For this review, take the finished solid that the model builds, in its own axes (mm). A direction names the side the tool comes from. Give positions to 0.01 mm unless a question says otherwise; leave off trailing zeros. Order: outer loops, then holes, each group sorted by start corner. A loop starts at its lowest first (then second) coordinate and runs counter-clockwise, first axis right, second up. Notation, with made-up numbers: (-6, 44) -> (12, 44) arc R16 ccw to (12, 65) -> close; hole circle Ø1 at (-18.75, 0.25). An arc over 180 degrees is marked (long way). Return JSON: item names as keys, results as strings. Group by question number.
1) Add section B-B (z = -94.5). Give the boundary of the cut face in (x, y), then the cut area to 3 significant figures.
2) Insertion check: P1, Ø3, axis at x = -9, y = 1.5, coming from the -Z side; P2, Ø2, axis at y = 4, z = -17, coming from the -X side; P3, Ø2.5, axis at x = -16.5, y = 3.5, coming from the +Z side. Each pin has a flat end and moves straight along its axis. Give the tip position at first contact, or say it passes through.
3) For faces 1 (the face through (-11, 2, 5)), 2 (the face through (6, 2, -78)), 3 (the face through (-8, 2, -80)), 4 (the face through (-23, 2, -180)), 5 (the face through (0, 3, -166)), list the 3-axis set-ups (+Z, -Z, +X, -X, +Y, -Y) from which the entire face can be reached by the end or side of a thin tool; tool diameter is ignored.
4) The part is to be moulded in two halves that separate along X. For faces 6 (the face through (9, 2, 5)), 7 (the face through (-19, 2, -160)), 8 (the face through (-17, 3, -173)), say which applies: released by +X, released by -X, zero draft, split by the parting line, or undercut.
5) Add section A-A (y = 3.3). Give the boundary of the cut face in (x, z), then the cut area to 3 significant figures.
6) To check wall thickness, follow line 1 along X through (y, z) = (2.6, -174); line 2 along X through (y, z) = (2.4, -170); line 3 along Z through (x, y) = (26, 1.6). State the ranges of each line that lie inside material, in increasing order.
from build123d import *

# Parameters (mm, degrees)
BOSS_EXTRUDE1_DEPTH = 5
SKETCH2_R           = 1.5
SKETCH2_W           = 32
SKETCH2_H           = 14
CUT_EXTRUDE1_DEPTH  = 10
FILLET1_R           = 2


with BuildPart() as part:
    # Sketch1 → Boss-Extrude1 (new body)
    with BuildSketch(Plane(origin=(0, 0, 0), x_dir=(1, 0, 0), z_dir=(0, 1, 0))):
        Polygon((9, -10), (9, 0), (6, 0), (6, 160), (28, 160), (28, 180), (-30, 180), (-30, 160), (-8, 160), (-8, 0), (-11, 0), (-11, -10), align=None)
    extrude(amount=BOSS_EXTRUDE1_DEPTH)

    # Sketch2 → Cut-Extrude1 (cut)
    with BuildSketch(Plane(origin=(0, 5, 0), x_dir=(1, 0, 0), z_dir=(0, 1, 0))):
        with Locations(Location((-21, 174, 0), (0, 0, 270))):
            Circle(SKETCH2_R)
        with Locations(Location((19, 174, 0), (0, 0, 270))):
            Circle(SKETCH2_R)
        with Locations((-1, 173)):
            Rectangle(SKETCH2_W, SKETCH2_H)
    extrude(amount=-CUT_EXTRUDE1_DEPTH, mode=Mode.SUBTRACT)

    # Fillet1
    fillet1_edges = [part.edges().sort_by_distance(p)[0] for p in [
        (-8, 2.5, -160),
        (-30, 2.5, -160),
        (-30, 2.5, -180),
        (28, 2.5, -180),
        (28, 2.5, -160),
        (6, 2.5, -160),
        (15, 2.5, -180),
        (-17, 2.5, -166),
        (-17, 2.5, -180),
    ]]
    fillet(fillet1_edges, radius=FILLET1_R)


solid = part.part
Evaluation:
{
 "1": {"outline": "(-8, 0) -> (6, 0) -> (6, 5) -> (-8, 5) -> close", "area": "70.0 mm^2"},
 "2": {"P1": "z = -166", "P2": "x = -8", "P3": "z = -160"},
 "3": {"face 1": "+Z, -X, +Y, -Y", "face 2": "+X, +Y, -Y", "face 3": "-X, +Y, -Y", "face 4": "-Z, +X, -X, +Y, -Y", "face 5": "-Z, +Y, -Y"},
 "4": {"face 6": "released by +X", "face 7": "zero draft", "face 8": "undercut"},
 "5": {"outline": "(-30, -178) arc R2 ccw to (-28, -180) -> (-19, -180) arc R2 ccw to (-17, -178) -> (-17, -168) arc R2 cw to (-15, -166) -> (15, -166) -> (15, -178) arc R2 ccw to (17, -180) -> (26, -180) arc R2 ccw to (28, -178) -> (28, -162) arc R2 ccw to (26, -160) -> (8, -160) arc R2 cw to (6, -158) -> (6, 0) -> (9, 0) -> (9, 10) -> (-11, 10) -> (-11, 0) -> (-8, 0) -> (-8, -158) arc R2 cw to (-10, -160) -> (-28, -160) arc R2 ccw to (-30, -162) -> close; hole circle Ø3 at (-21, -174); hole circle Ø3 at (19, -174)", "area": "3,140 mm^2"},
 "6": {"line 1": "-30 to -22.5, -19.5 to -17, 15 to 17.5, 20.5 to 28", "line 2": "-30 to -17, 15 to 28", "line 3": "-180 to -160"}
}
